from build123d import *

# Parameters (mm, degrees)
F1_DEPTH = 10
F2_DEPTH = 6
F3_DEPTH = 15
F0_W     = 7
F0_H     = 7
F4_DEPTH = 4
F5_DEPTH = 2


with BuildPart() as f1:
    # F0 (on Top) → F1 (new body)
    with BuildSketch(Plane.XY):
        with BuildLine():
            Line((26.5840129331, 34.7330055023), (-23.1406439107, 34.7330055023))
            Line((-23.1406439107, 34.7330055023), (-23.1406439107, 32.7330055023))
            ThreePointArc((-23.1406439107, 32.7330055023), (-21.7264303483, 32.1472190646), (-21.1406439107, 30.7330055023))
            Line((-21.1406439107, 30.7330055023), (-13.1406439107, 30.7330055023))
            Line((-13.1406439107, 30.7330055023), (12.5840129331, 30.7330055023))
            Line((12.5840129331, 30.7330055023), (20.5840129331, 30.7330055023))
            ThreePointArc((20.5840129331, 30.7330055023), (22.5840129331, 32.7330055023), (24.5840129331, 30.7330055023))
            ThreePointArc((24.5840129331, 30.7330055023), (23.9982264954, 29.3187919399), (22.5840129331, 28.7330055023))
            Line((22.5840129331, 28.7330055023), (22.5840129331, 20.7330055023))
            Line((22.5840129331, 20.7330055023), (22.5840129331, -35.2227493608))
            Line((22.5840129331, -35.2227493608), (22.5840129331, -43.2227493608))
            ThreePointArc((22.5840129331, -43.2227493608), (23.9982264954, -43.8085357985), (24.5840129331, -45.2227493608))
            Line((24.5840129331, -45.2227493608), (26.5840129331, -45.2227493608))
            Line((26.5840129331, -45.2227493608), (26.5840129331, 34.7330055023))
        make_face()
        with BuildLine():
            Line((-23.1406439107, 34.7330055023), (-27.1406439107, 34.7330055023))
            Line((-27.1406439107, 34.7330055023), (-27.1406439107, 30.7330055023))
            Line((-27.1406439107, 30.7330055023), (-25.1406439107, 30.7330055023))
            ThreePointArc((-25.1406439107, 30.7330055023), (-24.5548574731, 32.1472190646), (-23.1406439107, 32.7330055023))
            Line((-23.1406439107, 32.7330055023), (-23.1406439107, 34.7330055023))
        make_face()
        with BuildLine():
            Line((-25.1406439107, 30.7330055023), (-27.1406439107, 30.7330055023))
            Line((-27.1406439107, 30.7330055023), (-27.1406439107, -49.2227493608))
            Line((-27.1406439107, -49.2227493608), (22.5840129331, -49.2227493608))
            Line((22.5840129331, -49.2227493608), (22.5840129331, -47.2227493608))
            ThreePointArc((22.5840129331, -47.2227493608), (21.1697993707, -46.6369629232), (20.5840129331, -45.2227493608))
            Line((20.5840129331, -45.2227493608), (12.5840129331, -45.2227493608))
            Line((12.5840129331, -45.2227493608), (-13.1406439107, -45.2227493608))
            Line((-13.1406439107, -45.2227493608), (-21.1406439107, -45.2227493608))
            ThreePointArc((-21.1406439107, -45.2227493608), (-24.5548574731, -46.6369629232), (-23.1406439107, -43.2227493608))
            Line((-23.1406439107, -43.2227493608), (-23.1406439107, -35.2227493608))
            Line((-23.1406439107, -35.2227493608), (-23.1406439107, 20.7330055023))
            Line((-23.1406439107, 20.7330055023), (-23.1406439107, 28.7330055023))
            ThreePointArc((-23.1406439107, 28.7330055023), (-24.5548574731, 29.3187919399), (-25.1406439107, 30.7330055023))
        make_face()
        with BuildLine():
            Line((26.5840129331, -49.2227493608), (26.5840129331, -45.2227493608))
            Line((26.5840129331, -45.2227493608), (24.5840129331, -45.2227493608))
            ThreePointArc((24.5840129331, -45.2227493608), (23.9982264954, -46.6369629232), (22.5840129331, -47.2227493608))
            Line((22.5840129331, -47.2227493608), (22.5840129331, -49.2227493608))
            Line((22.5840129331, -49.2227493608), (26.5840129331, -49.2227493608))
        make_face()
    extrude(amount=F1_DEPTH)

    # F0 (on Top) → F2 (join)
    with BuildSketch(Plane.XY):
        with BuildLine():
            Line((-13.1406439107, 30.7330055023), (-21.1406439107, 30.7330055023))
            ThreePointArc((-21.1406439107, 30.7330055023), (-21.7264303483, 29.3187919399), (-23.1406439107, 28.7330055023))
            Line((-23.1406439107, 28.7330055023), (-23.1406439107, 20.7330055023))
            Line((-23.1406439107, 20.7330055023), (-20.1406439107, 20.7330055023))
            Line((-20.1406439107, 20.7330055023), (-20.1406439107, 27.7330055023))
            Line((-20.1406439107, 27.7330055023), (-13.1406439107, 27.7330055023))
            Line((-13.1406439107, 27.7330055023), (-13.1406439107, 30.7330055023))
        make_face()
        with BuildLine():
            Line((20.5840129331, 30.7330055023), (12.5840129331, 30.7330055023))
            Line((12.5840129331, 30.7330055023), (12.5840129331, 27.7330055023))
            Line((12.5840129331, 27.7330055023), (19.5840129331, 27.7330055023))
            Line((19.5840129331, 27.7330055023), (19.5840129331, 20.7330055023))
            Line((19.5840129331, 20.7330055023), (22.5840129331, 20.7330055023))
            Line((22.5840129331, 20.7330055023), (22.5840129331, 28.7330055023))
            ThreePointArc((22.5840129331, 28.7330055023), (21.1697993707, 29.3187919399), (20.5840129331, 30.7330055023))
        make_face()
        with BuildLine():
            ThreePointArc((20.5840129331, -45.2227493608), (21.1697993707, -43.8085357985), (22.5840129331, -43.2227493608))
            Line((22.5840129331, -43.2227493608), (22.5840129331, -35.2227493608))
            Line((22.5840129331, -35.2227493608), (19.5840129331, -35.2227493608))
            Line((19.5840129331, -35.2227493608), (19.5840129331, -42.2227493608))
            Line((19.5840129331, -42.2227493608), (12.5840129331, -42.2227493608))
            Line((12.5840129331, -42.2227493608), (12.5840129331, -45.2227493608))
            Line((12.5840129331, -45.2227493608), (20.5840129331, -45.2227493608))
        make_face()
        with BuildLine():
            Line((-20.1406439107, -35.2227493608), (-23.1406439107, -35.2227493608))
            Line((-23.1406439107, -35.2227493608), (-23.1406439107, -43.2227493608))
            ThreePointArc((-23.1406439107, -43.2227493608), (-21.7264303483, -43.8085357985), (-21.1406439107, -45.2227493608))
            Line((-21.1406439107, -45.2227493608), (-13.1406439107, -45.2227493608))
            Line((-13.1406439107, -45.2227493608), (-13.1406439107, -42.2227493608))
            Line((-13.1406439107, -42.2227493608), (-20.1406439107, -42.2227493608))
            Line((-20.1406439107, -42.2227493608), (-20.1406439107, -35.2227493608))
        make_face()
    extrude(amount=F2_DEPTH)

    # F0 (on Top) → F3 (join)
    with BuildSketch(Plane.XY):
        with BuildLine():
            Line((-21.1406439107, 30.7330055023), (-23.1406439107, 30.7330055023))
            Line((-23.1406439107, 30.7330055023), (-23.1406439107, 28.7330055023))
            ThreePointArc((-23.1406439107, 28.7330055023), (-21.7264303483, 29.3187919399), (-21.1406439107, 30.7330055023))
        make_face()
        with BuildLine():
            Line((-23.1406439107, 30.7330055023), (-23.1406439107, 32.7330055023))
            ThreePointArc((-23.1406439107, 32.7330055023), (-24.5548574731, 32.1472190646), (-25.1406439107, 30.7330055023))
            Line((-25.1406439107, 30.7330055023), (-23.1406439107, 30.7330055023))
        make_face()
        with BuildLine():
            ThreePointArc((-21.1406439107, 30.7330055023), (-21.7264303483, 32.1472190646), (-23.1406439107, 32.7330055023))
            Line((-23.1406439107, 32.7330055023), (-23.1406439107, 30.7330055023))
            Line((-23.1406439107, 30.7330055023), (-21.1406439107, 30.7330055023))
        make_face()
        with BuildLine():
            Line((-23.1406439107, 30.7330055023), (-25.1406439107, 30.7330055023))
            ThreePointArc((-25.1406439107, 30.7330055023), (-24.5548574731, 29.3187919399), (-23.1406439107, 28.7330055023))
            Line((-23.1406439107, 28.7330055023), (-23.1406439107, 30.7330055023))
        make_face()
        with BuildLine():
            ThreePointArc((24.5840129331, 30.7330055023), (22.5840129331, 32.7330055023), (20.5840129331, 30.7330055023))
            Line((20.5840129331, 30.7330055023), (22.5840129331, 30.7330055023))
            Line((22.5840129331, 30.7330055023), (22.5840129331, 28.7330055023))
            ThreePointArc((22.5840129331, 28.7330055023), (23.9982264954, 29.3187919399), (24.5840129331, 30.7330055023))
        make_face()
        with BuildLine():
            Line((22.5840129331, 30.7330055023), (20.5840129331, 30.7330055023))
            ThreePointArc((20.5840129331, 30.7330055023), (21.1697993707, 29.3187919399), (22.5840129331, 28.7330055023))
            Line((22.5840129331, 28.7330055023), (22.5840129331, 30.7330055023))
        make_face()
        with BuildLine():
            Line((20.5840129331, -45.2227493608), (22.5840129331, -45.2227493608))
            Line((22.5840129331, -45.2227493608), (22.5840129331, -43.2227493608))
            ThreePointArc((22.5840129331, -43.2227493608), (21.1697993707, -43.8085357985), (20.5840129331, -45.2227493608))
        make_face()
        with BuildLine():
            Line((22.5840129331, -45.2227493608), (24.5840129331, -45.2227493608))
            ThreePointArc((24.5840129331, -45.2227493608), (23.9982264954, -43.8085357985), (22.5840129331, -43.2227493608))
            Line((22.5840129331, -43.2227493608), (22.5840129331, -45.2227493608))
        make_face()
        with BuildLine():
            ThreePointArc((22.5840129331, -47.2227493608), (23.9982264954, -46.6369629232), (24.5840129331, -45.2227493608))
            Line((24.5840129331, -45.2227493608), (22.5840129331, -45.2227493608))
            Line((22.5840129331, -45.2227493608), (22.5840129331, -47.2227493608))
        make_face()
        with BuildLine():
            ThreePointArc((20.5840129331, -45.2227493608), (21.1697993707, -46.6369629232), (22.5840129331, -47.2227493608))
            Line((22.5840129331, -47.2227493608), (22.5840129331, -45.2227493608))
            Line((22.5840129331, -45.2227493608), (20.5840129331, -45.2227493608))
        make_face()
        with BuildLine():
            ThreePointArc((-21.1406439107, -45.2227493608), (-21.7264303483, -43.8085357985), (-23.1406439107, -43.2227493608))
            Line((-23.1406439107, -43.2227493608), (-23.1406439107, -45.2227493608))
            Line((-23.1406439107, -45.2227493608), (-21.1406439107, -45.2227493608))
        make_face()
        with BuildLine():
            Line((-23.1406439107, -45.2227493608), (-23.1406439107, -43.2227493608))
            ThreePointArc((-23.1406439107, -43.2227493608), (-24.5548574731, -46.6369629232), (-21.1406439107, -45.2227493608))
            Line((-21.1406439107, -45.2227493608), (-23.1406439107, -45.2227493608))
        make_face()
    extrude(amount=F3_DEPTH)

    # F0 (on Top) → F4 (join)
    with BuildSketch(Plane.XY):
        with Locations((-16.6406439107, 24.2330055023)):
            Rectangle(F0_W, F0_H)
        with Locations((16.0840129331, 24.2330055023)):
            Rectangle(F0_W, F0_H)
        with Locations((16.0840129331, -38.7227493608)):
            Rectangle(F0_W, F0_H)
        with Locations((-16.6406439107, -38.7227493608)):
            Rectangle(F0_W, F0_H)
    extrude(amount=F4_DEPTH)

    # F0 (on Top) → F5 (join)
    with BuildSketch(Plane.XY):
        Polygon((12.5840129331, 30.7330055023), (-13.1406439107, 30.7330055023), (-13.1406439107, 27.7330055023), (-13.1406439107, 20.7330055023), (-20.1406439107, 20.7330055023), (-23.1406439107, 20.7330055023), (-23.1406439107, -35.2227493608), (-20.1406439107, -35.2227493608), (-13.1406439107, -35.2227493608), (-13.1406439107, -42.2227493608), (-13.1406439107, -45.2227493608), (12.5840129331, -45.2227493608), (12.5840129331, -42.2227493608), (12.5840129331, -35.2227493608), (19.5840129331, -35.2227493608), (22.5840129331, -35.2227493608), (22.5840129331, 20.7330055023), (19.5840129331, 20.7330055023), (12.5840129331, 20.7330055023), (12.5840129331, 27.7330055023), align=None)
    extrude(amount=F5_DEPTH)


solid = f1.part
Input: part model. Units: mm. Frame: model coordinates. A direction names the side the tool comes from. Coordinates: 2 decimals unless noted, no trailing zeros. Loops run counter-clockwise (first coordinate to the right, second up) from the corner with the lowest first, then second, coordinate; pieces in that order, holes last.
(1) Section C-C on y = 24.5. Return the cut outline in (x, z), then the cut area to 3 significant figures.
(2) Section B-B on z = 7. Return the cut outline in (x, y).
(3) Set-up query: faces 4 (the face through (-1, -7, 0)), 5 (the face through (16, 24, 4)). Return all of +Z, -Z, +X, -X, +Y, -Y with unobstructed straight access to the full face (end or side cutting, diameter ignored); none if empty.
(4) Pull-direction query (X, two-part tool) for faces 1 (the face through (26.584, -8, 5)), 2 (the face through (16, -42.223, 5)), 3 (the face through (23, 31, 15)); classes: released by +X, released by -X, zero draft, split by the parting line, or undercut.
(5) First-contact query: pin 1 Ø2 at (x, y) = (17, 22.5) entering from +Z; pin 2 Ø10 at (x, y) = (-8.5, -22.5) entering from +Z. Flat tips, straight axial feed; report the tip coordinate or a pass-through.
(6) Section A-A on z = 13. Return the cut outline in (x, y).
(7) Section D-D on x = -6. Return the cut outline in (y, z), then the cut area to 3 significant figures.
(8) Material intervals for probe 1 along Y at (x, z) = (-20.5, 5.5); probe 2 along X at (y, z) = (-7, 5); probe 3 along Y at (x, z) = (-0.5, 2.25), sorted ascending.
Data:
1. outline: (-27.14, 0) - (26.58, 0) - (26.58, 10) - (22.58, 10) - (22.58, 6) - (19.58, 6) - (19.58, 4) - (12.58, 4) - (12.58, 2) - (-13.14, 2) - (-13.14, 4) - (-20.14, 4) - (-20.14, 6) - (-23.14, 6) - (-23.14, 10) - (-27.14, 10) - close
1. area: 223 mm2
2. outline: (-27.14, -49.22) - (26.58, -49.22) - (26.58, 34.73) - (-27.14, 34.73) - close; hole (-23.14, -43.22) arc R2 cw to (-21.14, -45.22) - (20.58, -45.22) arc R2 cw to (22.58, -43.22) - (22.58, 28.73) arc R2 cw to (20.58, 30.73) - (-21.14, 30.73) arc R2 cw to (-23.14, 28.73) - close
3. face 4: -Z, +X, -X, +Y, -Y
3. face 5: +Z
4. face 1: released by +X
4. face 2: undercut
4. face 3: zero draft
5. pin 1: stops at z = 4
5. pin 2: stops at z = 2
6. outline: circle Ø4 at (-23.14, -45.22); circle Ø4 at (-23.14, 30.73); circle Ø4 at (22.58, -45.22); circle Ø4 at (22.58, 30.73)
7. outline: (-49.22, 0) - (34.73, 0) - (34.73, 10) - (30.73, 10) - (30.73, 2) - (-45.22, 2) - (-45.22, 10) - (-49.22, 10) - close
7. area: 232 mm2
8. probe 1: y = -49.22 to -35.22, 20.73 to 34.73
8. probe 2: x = -27.14 to -23.14, 22.58 to 26.58
8. probe 3: y = -49.22 to -45.22, 30.73 to 34.73
